The model under review builds one solid part; all positions refer to its coordinate system, in mm. A direction names the side the tool comes from. Coordinates: 2 decimals unless noted, no trailing zeros. Loops run counter-clockwise (first coordinate to the right, second up) from the corner with the lowest first, then second, coordinate; pieces in that order, holes last. Notation, with made-up numbers: (11, -18) - (19, -18) arc R18 ccw to (19, 13) - close; hole circle Ø4 at (26.5, 55.25). An arc over 180 degrees is marked (long way). Answer in a Markdown table with one row per item. Add a question column.
(1) Mouldability with a two-part tool opening along X and no side actions: class faces 1 (the cylindrical face through (12.557, 2.923, -3.042)), 2 (the cylindrical face through (2.6, -4.99, -2.96)), 3 (the flat face through (1, 12.25, -4)) as +X half, -X half, draft (parallel to the pull), parting line (faces both ways), or undercut.
(2) We need section B-B on y = 8. Write out the cut boundary in (x, z).
(3) For line 1 along Y through (x, z) = (0, -3.5) (3 decimals); line 2 along Y through (x, z) = (-1, -2); line 3 along Z through (x, y) = (32.5, 9), list the stretches that pass through material, from the lowest coordinate up.
(4) Machinability: for faces 4 (the cylindrical face through (-0.19, 11.25, -7.97)), 5 (the cylindrical face through (31.19, 8.19, -5)), which of the approach directions +Z, -Z, +X, -X, +Y, -Y give a long, thin tool a straight path to every point of the face, cutting with its end or side? Answer none if there is none.
(5) We need section D-D on x = 21.5. Write out the cut boundary in (y, z), plus the area to 3 significant figures.
(6) We need section C-C on z = -7.25. Write out the cut boundary in (x, y).
(7) For P1, Ø3, axis at x = 30, z = -7.5, coming from the -Y side; P2, Ø5.5, axis at x = 17.5, z = -4, coming from the -Y side; P3, Ø0.9, axis at x = -2.5, y = 14.5, coming from the +Z side, all flat-tipped, find the tip position at first contact; note any pin that passes through.
(8) We need section A-A on x = -32.5. Write out the cut boundary in (y, z), plus the area to 3 significant figures.
from build123d import *

# Parameters (mm, degrees)
F4_D      = 2.5
F3_R      = 5.625
F5_DEPTH  = 18.001
F7_DEPTH  = 10
F8_R      = 4.5
F9_W      = 80
F9_H      = 2
F10_DEPTH = 3
F12_D     = 3.3


with BuildPart() as f1:
    # F0 (on Front) → F1 (revolve)
    with BuildSketch(Plane.XZ):
        Polygon((5.125, 1.85), (3.5, 1.85), (3.5, -16.15), (5.125, -16.15), (5.125, -6), (11.25, -6), (11.25, 0), (5.125, 0), align=None)
    revolve(axis=Axis((0, 0, -12.1311874992), (0, 0, -1)))

    # F4 (through all)
    with Locations(Plane.XY):
        with Locations((0, 8), (8, 0), (0, -8), (-8, 0)):
            Hole(F4_D / 2)

    # F3 (on face) → F5 (cut, through all)
    with BuildSketch(Plane.XY.offset(1.85)):
        Circle(F3_R)
    extrude(amount=-F5_DEPTH, mode=Mode.SUBTRACT)

    # F6 (on face) → F7 (join)
    with BuildSketch(Plane.XY):
        with BuildLine():
            ThreePointArc((-10.416333328, 4.25), (0, 11.25), (10.416333328, 4.25))
            Line((10.416333328, 4.25), (40, 4.25))
            Line((40, 4.25), (40, 12.25))
            Line((40, 12.25), (-40, 12.25))
            Line((-40, 12.25), (-40, 4.25))
            Line((-40, 4.25), (-10.416333328, 4.25))
        make_face()
    extrude(amount=-F7_DEPTH)

    # F8
    f8_edges = [f1.edges().sort_by_distance(p)[0] for p in [
        (10.416333, 4.25, -3),
        (-10.416333, 4.25, -3),
    ]]
    fillet(f8_edges, radius=F8_R)

    # F9 (on face) → F10 (join)
    with BuildSketch(Plane(origin=(0, 12.25, 0), x_dir=(-1, 0, 0), z_dir=(0, 1, 0))):
        with Locations((0, -9)):
            Rectangle(F9_W, F9_H)
    extrude(amount=F10_DEPTH)

    # F12 (through all)
    with Locations(Plane(origin=(0, 12.25, 0), x_dir=(-1, 0, 0), z_dir=(0, 1, 0))):
        with Locations((-32.5, -4), (-17.5, -4), (17.5, -4), (32.5, -4)):
            Hole(F12_D / 2)


solid = f1.part
Outcome:
| question | item | result |
|---|---|---|
| 1 | face 1 | +X half |
| 1 | face 2 | undercut |
| 1 | face 3 | draft |
| 2 | outline | (-40, -10) - (-7.91, -10) - (-7.91, -6) - (-1.25, -6) - (-1.25, 0) - (-40, 0) - close; (1.25, -6) - (7.91, -6) - (7.91, -10) - (40, -10) - (40, 0) - (1.25, 0) - close; hole circle Ø3.3 at (-32.5, -4); hole circle Ø3.3 at (-17.5, -4); hole circle Ø3.3 at (17.5, -4); hole circle Ø3.3 at (32.5, -4) |
| 3 | line 1 | -11.25 to -9.25, -6.75 to -5.625, 5.625 to 6.75, 9.25 to 12.25 |
| 3 | line 2 | -11.21 to -8.75, -7.25 to -5.54, 5.54 to 7.25, 8.75 to 12.25 |
| 3 | line 3 | -10 to -5.65, -2.35 to 0 |
| 4 | face 4 | -Z, -Y |
| 4 | face 5 | +Y, -Y |
| 5 | outline | (4.25, -10) - (15.25, -10) - (15.25, -8) - (12.25, -8) - (12.25, 0) - (4.25, 0) - close |
| 5 | area | 86.0 mm² |
| 6 | outline | (-40, 4.25) - (-10.42, 4.25) arc R11.25 cw to (10.42, 4.25) - (40, 4.25) - (40, 12.25) - (-40, 12.25) - close |
| 7 | P1 | y = 4.25 |
| 7 | P2 | y = 4.14 |
| 7 | P3 | z = -8 |
| 8 | outline | (4.25, -10) - (15.25, -10) - (15.25, -8) - (12.25, -8) - (12.25, -5.65) - (4.25, -5.65) - close; (4.25, -2.35) - (12.25, -2.35) - (12.25, 0) - (4.25, 0) - close |
| 8 | area | 59.6 mm² |
